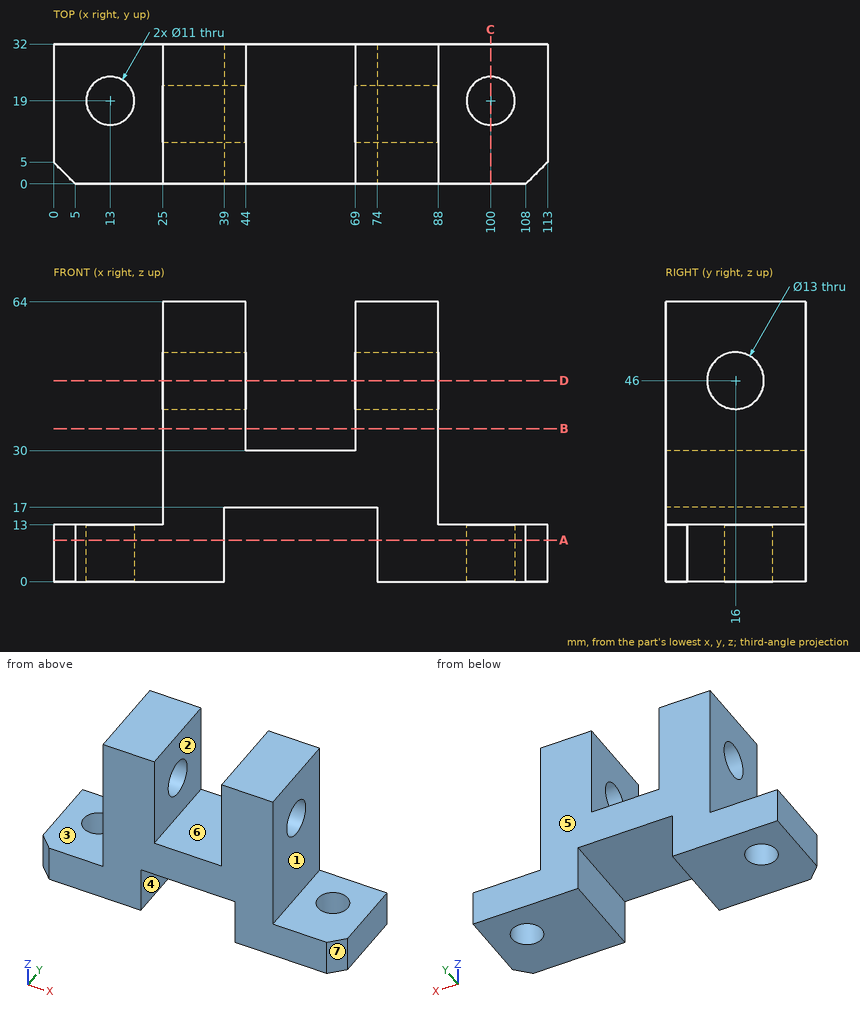
For this review, use the dimensioned drawing (mm, ordinates from the lowest corner) and the shaded views. A direction names the side the tool comes from. Give positions to 0.01 mm unless a question says otherwise; leave off trailing zeros. Loops run counter-clockwise (first coordinate to the right, second up) from the corner with the lowest first, then second, coordinate; pieces in that order, holes last.
Item 1: Take a section at C-C, the plane x = 100. State the section outline as (y, z) points, and give its area (3 significant figures).
Item 2: Draft analysis for pull direction X (two halves, no side actions). For the marked faces 5, 6 and 7, state which applies: +X half, -X half, draft (parallel to the pull), parting line (faces both ways), or undercut.
Item 3: Take a section at D-D, the plane z = 46. State the section outline as (x, y) points.
Item 4: Take a section at A-A, the plane z = 9.5. State the section outline as (x, y) points.
Item 5: Take a section at B-B, the plane z = 35. State the section outline as (x, y) points.
Item 6: For line 1 along Z through (x, y) = (40.25, 16); line 2 along X through (y, z) = (28, 43.5); line 3 along Y through (x, z) = (13, 6), list the stretches that pass through material, from the lowest coordinate up.
Item 7: Insertion check: pin 1 (7.5 mm diameter, centred on x = 104, y = 13.5, fed in from +Z); pin 2 (6.5 mm diameter, centred on x = 100, y = 19, fed in from +Z); pin 3 (12.5 mm diameter, centred on x = 59, y = 12.5, fed in from +Z); pin 4 (16 mm diameter, centred on y = 12, z = 33.5, fed in from +X). Each pin has a flat end and moves straight along its axis. Give the tip position at first contact, or say it passes through.
Item 8: Tool access review of the marked faces 1, 2, 3 and 4: name each direction out of +Z, -Z, +X, -X, +Y, -Y from which nothing blocks a thin tool from reaching the whole face with its end or side.
Calculated:
1. outline: (0, 0) - (13.5, 0) - (13.5, 13) - (0, 13) - close; (24.5, 0) - (32, 0) - (32, 13) - (24.5, 13) - close
1. area: 273 mm2
2. face 5: draft
2. face 6: undercut
2. face 7: +X half
3. outline: (25, 0) - (44, 0) - (44, 9.5) - (25, 9.5) - close; (25, 22.5) - (44, 22.5) - (44, 32) - (25, 32) - close; (69, 0) - (88, 0) - (88, 9.5) - (69, 9.5) - close; (69, 22.5) - (88, 22.5) - (88, 32) - (69, 32) - close
4. outline: (0, 5) - (5, 0) - (39, 0) - (39, 32) - (0, 32) - close; (74, 0) - (108, 0) - (113, 5) - (113, 32) - (74, 32) - close; hole circle Ø11 at (13, 19); hole circle Ø11 at (100, 19)
5. outline: (25, 0) - (44, 0) - (44, 32) - (25, 32) - close; (69, 0) - (88, 0) - (88, 32) - (69, 32) - close
6. line 1: z = 17 to 39.5, 52.5 to 64
6. line 2: x = 25 to 44, 69 to 88
6. line 3: y = 0 to 13.5, 24.5 to 32
7. pin 1: stops at z = 13
7. pin 2: passes through
7. pin 3: stops at z = 30
7. pin 4: stops at x = 88
8. face 1: +Z, +X, +Y, -Y
8. face 2: +Z, +Y, -Y
8. face 3: +Z, -X, +Y, -Y
8. face 4: -Z, +Y, -Y
